Could you check a few things on this model? Use its own coordinates, in mm. A direction names the side the tool comes from. Round coordinates to 2 decimals unless told otherwise and drop trailing zeros. Loops run counter-clockwise (first coordinate to the right, second up) from the corner with the lowest first, then second, coordinate; pieces in that order, holes last. Notation, with made-up numbers: (71.5, 23.5) -> (93.5, 23.5) arc R31 ccw to (93.5, 60.5) -> close; hole circle Ø11 at (-27.75, 55.25). An arc over 180 degrees is marked (long way). One line per item, written item: value.
Autodesk Inventor part; units mm, degrees
ref_plane "YZ Plane" through (0, 0, 0) normal (1, 0, 0) x (0, 1, 0)
ref_plane "XZ Plane" through (0, 0, 0) normal (0, 1, 0) x (-1, 0, 0)
ref_plane "XY Plane" through (0, 0, 0) normal (0, 0, 1) x (1, 0, 0)
sketch "Sketch1" plane through (0, 0, 0) normal (0, 0, 1) x (1, 0, 0)
  line L0 (-19.520958, 8.240943) -> (7.466542, 8.240943)
  line L1 (7.466542, 8.240943) -> (7.466542, -9.221557)
  line L2 (7.466542, -9.221557) -> (-19.520958, -9.221557)
  line L3 (-19.520958, -9.221557) -> (-19.520958, 8.240943)
  point P0 (0, 0)
  dimension "d0" = 17.4625
  dimension "d1" = 26.9875
extrude "Extrusion1" add sketch "Sketch1" along normal blind 1.5875
sketch "Sketch2" plane through (0, 0, 1.5875) normal (0, 0, 1) x (1, 0, 0)
  line L0 (7.466542, 8.240943) -> (7.466542, -9.221557)
  line L1 (7.466542, -9.221557) -> (-19.520958, -9.221557)
  circle A0 centre (4.291542, -4.459057) radius 3.175
  point P0 (0, 0)
  dimension "d4" = 4.7625
  dimension "d5" = 6.35
extrude "Extrusion2" add sketch "Sketch2" along normal blind 6.35
fillet "Fillet1" radius 0.635 1 edges at (1.1165, -4.4591, 7.9375)
sketch "Sketch3" plane through (0, 0, 1.5875) normal (0, 0, 1) x (1, 0, 0)
  line L0 (0.379367, 7.296145) -> (6.490253, 7.296145)
  line L1 (6.490253, 7.296145) -> (6.490253, 2.269448)
  line L2 (6.490253, 2.269448) -> (0.379367, 2.269448)
  line L3 (0.379367, 2.269448) -> (0.379367, 7.296145)
  point P0 (0, 0)
extrude "Extrusion3" add sketch "Sketch3" along normal blind 3.175
sketch "Sketch4" plane through (7.466542, -9.221557, 0) normal (1, 0, 0) x (0, 0, -1)
  line L0 (-1.5875, 17.4625) -> (-1.5875, 4.7625)
  line L1 (-1.5875, 4.7625) -> (-1.5875, 0)
  line L2 (0, 0) -> (-1.5875, 0)
  line L3 (0, 17.4625) -> (0, 0)
  line L4 (0, 17.4625) -> (-1.5875, 17.4625)
  circle A0 centre (-0.79375, 16.66875) radius 0.79375
  circle A1 centre (-0.79375, 0.79375) radius 0.79375
  circle A2 centre (-0.79375, 8.73125) radius 0.15875
  circle A3 centre (-0.79375, 9.04875) radius 0.15875
  circle A4 centre (-0.79375, 8.41375) radius 0.15875
  line L5 (-0.79375, 0.79375) -> (-0.79375, 16.66875) construction
  line L6 (-0.79375, 0.79375) -> (-0.79375, 8.73125) construction
  line L7 (-0.79375, 8.73125) -> (-0.79375, 16.66875) construction
  point P0 (0, 9.221557)
  dimension "d11" = 0.3175
extrude "Extrusion4" add sketch "Sketch4" along normal blind 0.254 contours A0 | A1 | A2 | A4 | A3
sketch "Sketch5" plane through (-19.520958, -9.221557, 0) normal (-1, 0, 0) x (0, 0, 1)
  line L0 (1.5875, 0) -> (1.5875, 17.4625)
  line L1 (0, 17.4625) -> (1.5875, 17.4625)
  line L2 (0, 0) -> (0, 17.4625)
  line L3 (0, 0) -> (1.5875, 0)
  circle A0 centre (0.79375, 16.66875) radius 0.79375
  circle A1 centre (0.79375, 8.73125) radius 0.79375
  circle A2 centre (0.79375, 0.79375) radius 0.79375
  line L4 (0.79375, 16.66875) -> (0.79375, 8.73125) construction
  line L5 (0.79375, 0.79375) -> (0.79375, 8.73125) construction
  point P0 (0, 9.221557)
extrude "Extrusion5" add sketch "Sketch5" along normal blind 0.254 contours A2 | A1 | A0
sketch "Sketch6" plane through (7.720542, -8.427807, 0.79375) normal (1, 0, 0) x (0, 0, -1)
  circle A0 centre (0, 0) radius 0.79375 construction
sketch "Sketch7" plane through (7.720542, -0.172807, 0.79375) normal (1, 0, 0) x (0, 0, -1)
  circle A0 centre (0, 0) radius 0.15875 construction
  point P0 (0, -0.15875)
sketch "Sketch8" plane through (7.720542, -9.221557, 0) normal (1, 0, 0) x (0, 0, -1)
  arc A0 (-0.79375, 8.5725) -> (-0.79375, 8.89) centre (-0.79375, 8.73125) ccw construction
sketch "Sketch9" plane through (7.720542, -0.807807, 0.79375) normal (1, 0, 0) x (0, 0, -1)
  circle A0 centre (0, 0) radius 0.15875 construction
  point P0 (0, 0.15875)
sketch "Sketch10" plane through (-19.774958, 7.447193, 0.79375) normal (-1, 0, 0) x (0, 0, 1)
  circle A0 centre (0, 0) radius 0.79375 construction
sketch "Sketch11" plane through (-19.774958, -0.490307, 0.79375) normal (-1, 0, 0) x (0, 0, 1)
  circle A0 centre (0, 0) radius 0.79375 construction
sketch "Sketch12" plane through (-19.774958, -8.427807, 0.79375) normal (-1, 0, 0) x (0, 0, 1)
  circle A0 centre (0, 0) radius 0.79375 construction
properties part number "ESC"
(1) Imagine slicing it at C-C on x = -4.5. Write out the boundary of the cut face in (y, z).
Results below:
outline: (-9.22, 0) -> (8.24, 0) -> (8.24, 1.59) -> (-9.22, 1.59) -> close
(2) We'd pull the mould along Y, two halves only. Please class faces 1 (the face through (7.721, 7, 1)), 2 (the face through (-6, 8.241, 1)), 3 (the face through (-19.521, -5, 1)): +Y half, -Y half, draft (parallel to the pull), parting line (faces both ways), or undercut.
Results below:
face 1: draft
face 2: +Y half
face 3: undercut
(3) Imagine slicing it at B-B on y = 2. Write out the boundary of the cut face in (x, z), then the cut area to 3 significant figures.
Results below:
outline: (-19.52, 0) -> (7.47, 0) -> (7.47, 1.59) -> (-19.52, 1.59) -> close
area: 42.8 mm²
(4) Imagine slicing it at A-A on z = 4. Write out the boundary of the cut face in (x, y) (3 decimals).
Results below:
outline: (0.379, 2.269) -> (6.49, 2.269) -> (6.49, 7.296) -> (0.379, 7.296) -> close; circle Ø6.35 at (4.292, -4.459)
(5) On a 3-axis mill with a long thin cutter (end or side, diameter ignored), from which of +Z, -Z, +X, -X, +Y, -Y can I reach the whole of each face in a straight line? I mean faces 4 (the face through (3.6, -1.36, 4.4)), 5 (the face through (3, 2.269, 3)), 6 (the face through (3, 5, 4.762)), 7 (the face through (6.49, 5, 3)). Say none if no direction works.
Results below:
face 4: +Z
face 5: +Z, +X, -X
face 6: +Z, +X, -X, +Y
face 7: +Z, +X, +Y
(6) Imagine slicing it at D-D on z = 5.75. Write out the boundary of the cut face in (x, y) (3 decimals), then the cut area to 3 significant figures.
Results below:
outline: circle Ø6.35 at (4.292, -4.459)
area: 31.7 mm²
(7) Please list where these lines run through material, in increasing order: L1, parallel to Z at x = 5.75, y = -8; L2, parallel to X at y = -5, z = 1.25; L3, parallel to X at y = 4.5, z = 4.
Results below:
L1: z = 0 to 1.59
L2: x = -19.52 to 7.47
L3: x = 0.38 to 6.49
(8) For pin 1 Ø1.5 at (x, y) = (-9.5, -5) entering from +Z; pin 2 Ø2 at (x, z) = (-5.5, 4.5) entering from +Y; pin 3 Ø2.5 at (y, z) = (4.5, 3.5) entering from -X; pin 4 Ø1.3 at (y, z) = (-2.5, 1) entering from -X, each with a flat end and sliding along its axis, tell me the tip position at first contact or that it passes through.
Results below:
pin 1: stops at z = 1.59
pin 2: passes through
pin 3: stops at x = 0.38
pin 4: stops at x = -19.52
